Solid Edge part; units mm, degrees
sketch "Sketch1" plane through (0, 0, 0) normal (0, 0, 1) x (1, 0, 0)
  circle A0 centre (-10, 0) radius 5.15
  circle A1 centre (-10, 0) radius 10
extrude "Protrusion1" add sketch "Sketch1" along normal blind 9
sketch "Sketch2" plane through (0, 0, 0) normal (1, 0, 0) x (0, 1, 0)
  circle A0 centre (0, 4.5) radius 1.65
extrude "ExtrudedCutout_1" cut sketch "Sketch2" along normal mid plane 46.3227
sketch "Sketch3" plane through (0, 0, 0) normal (1, 0, 0) x (0, 1, 0)
  line L0 (2.9, 2.8257) -> (2.9, 6.1743)
  line L1 (2.9, 6.1743) -> (0, 7.8486)
  line L2 (0, 7.8486) -> (-2.9, 6.1743)
  line L3 (-2.9, 6.1743) -> (-2.9, 2.8257)
  line L4 (-2.9, 2.8257) -> (0, 1.1514)
  line L5 (0, 1.1514) -> (2.9, 2.8257)
extrude "ExtrudedCutout_2" cut sketch "Sketch3" along normal mid plane 5.5
Geometry: final body of the model. Coordinates: model frame, mm. A direction names the side the tool comes from. Give positions to 0.01 mm unless a question says otherwise; leave off trailing zeros. Order: outer loops, then holes, each group sorted by start corner. A loop starts at its lowest first (then second) coordinate and runs counter-clockwise, first axis right, second up. Notation, with made-up numbers: M 75.5,13 L 115.5,13 A6 cw 115.5,21 Z; hole C -36.75,40.5 d1. An arc over 180 degrees is marked long. Answer as CSV lines item,"result". Start each with the question number.
1) Cut plane C-C (y = 3.5). Output: boundary loops of the cut face in (x, z), then the cut area to 3 significant figures.
2) Cut plane D-D (x = -3). Output: boundary loops of the cut face in (y, z), then the cut area to 3 significant figures.
3) Line query: line 1 (Z direction, x = -3.5, y = 0); line 2 (X direction, y = -3.25, z = 4.5) (3 decimals); line 3 (Y direction, x = -16.35, z = 4.5). Output: solid intervals per line, ascending. Write a range as from..to.
4) First-contact query: P1, Ø3, axis at y = 8, z = 6, coming from the -X side; P2, Ø1, axis at y = 3.5, z = 5, coming from the -X side; P3, Ø1.5, axis at x = -2.5, z = 5.5, coming from the +Y side; P4, Ø3, axis at y = 0, z = 4.5, coming from the +X side. Flat tips, straight axial feed; report the tip coordinate or a pass-through.
5) Cut plane B-B (z = 4.5). Output: boundary loops of the cut face in (x, y).
6) Set-up query: faces 4 (the flat face through (-15, 2, 0)), 5 (the flat face through (-1.39, 1.47, 7)). Return all of +Z, -Z, +X, -X, +Y, -Y with unobstructed straight access to the full face (end or side cutting, diameter ignored); none if empty.
7) Cut plane A-A (x = -10). Output: boundary loops of the cut face in (y, z), then the cut area to 3 significant figures.
8) Mould query, pull axis Y, two halves, no side actions, for faces 1 (the cylindrical face through (-3.92, -1.65, 4.57)), 2 (the flat face through (-15, 2, 9)), 3 (the cylindrical face through (-0.763, 3.83, 4.437)). Classes: +Y half, -Y half, draft (parallel to the pull), parting line (faces both ways), or undercut.
Findings below:
1,outline,"M -19.37,0 L -13.78,0 L -13.78,9 L -19.37,9 Z; M -6.22,0 L -0.63,0 L -0.63,9 L -6.22,9 Z"
1,area,"101 mm²"
2,outline,"M -7.14,0 L 7.14,0 L 7.14,9 L -7.14,9 Z; hole C 0,4.5 d3.3"
2,area,"120 mm²"
3,line 1,"z = 0..2.85, 6.15..9"
3,line 2,"x = -19.457..-13.995, -6.005..-0.543"
3,line 3,"y = -7.73..-1.65, 1.65..7.73"
4,P1,"stops at x = -17.6"
4,P2,"stops at x = -19.54"
4,P3,"stops at y = 7.38"
4,P4,"passes through"
5,outline,"M -19.86,-1.65 A10 ccw -0.43,-2.9 L -2.75,-2.9 L -2.75,-1.65 L -5.12,-1.65 A5.15 cw -14.88,-1.65 Z; M -19.86,1.65 L -14.88,1.65 A5.15 cw -5.12,1.65 L -2.75,1.65 L -2.75,2.9 L -0.43,2.9 A10 ccw Z"
6,face 4,"-Z, +X, -X, +Y, -Y"
6,face 5,"+X"
7,outline,"M -10,0 L -5.15,0 L -5.15,9 L -10,9 Z; M 5.15,0 L 10,0 L 10,9 L 5.15,9 Z"
7,area,"87.3 mm²"
8,face 1,"undercut"
8,face 2,"draft"
8,face 3,"parting line"
